from build123d import *

# Parameters (mm, degrees)
SKETCH_1_W      = 38.4
SKETCH_1_H      = 54.1
EXTRUDE_1_DEPTH = 0.8
SKETCH_2_W      = 10
SKETCH_2_H      = 10
EXTRUDE_2_DEPTH = 3


with BuildPart() as part:
    # Эскиз1 → Бобышка-Вытянуть1 (new, symmetric)
    with BuildSketch(Plane(origin=(0, 0, 0), x_dir=(1, 0, 0), z_dir=(0, 1, 0))):
        Rectangle(SKETCH_1_W, SKETCH_1_H)
    extrude(amount=EXTRUDE_1_DEPTH, both=True)

    # Эскиз2 → Бобышка-Вытянуть2 (add)
    with BuildSketch(Plane(origin=(0, 0.8, 0), x_dir=(1, 0, 0), z_dir=(0, 1, 0))):
        with Locations((-14.2, 19.164621175)):
            Rectangle(SKETCH_2_W, SKETCH_2_H)
        with Locations((-14.2, 6.274815906)):
            Rectangle(SKETCH_2_W, SKETCH_2_H)
        with Locations((-14.2, -7.606512846)):
            Rectangle(SKETCH_2_W, SKETCH_2_H)
        with Locations((-14.2, -20.685179731)):
            Rectangle(SKETCH_2_W, SKETCH_2_H)
        with Locations((14.2, 18.692467136)):
            Rectangle(SKETCH_2_W, SKETCH_2_H)
        with Locations((14.2, 5.897092674)):
            Rectangle(SKETCH_2_W, SKETCH_2_H)
        with Locations((14.2, -6.756635575)):
            Rectangle(SKETCH_2_W, SKETCH_2_H)
        with Locations((14.2, -21.110118366)):
            Rectangle(SKETCH_2_W, SKETCH_2_H)
    extrude(amount=EXTRUDE_2_DEPTH)


solid = part.part
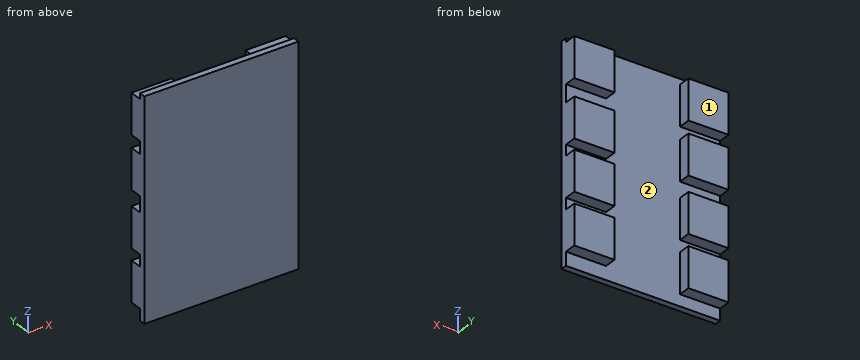
Build history of the part. All positions in model axes, mm. Face numbers are marked on the shaded views. Round coordinates to 2 decimals unless told otherwise and drop trailing zeros. Loops run counter-clockwise (first coordinate to the right, second up) from the corner with the lowest first, then second, coordinate; pieces in that order, holes last. Notation, with made-up numbers: (-24, -18.75) -> (13, -18.75) arc R25 cw to (13, 5.25) -> close; hole circle Ø9 at (37.25, -6). An arc over 180 degrees is marked (long way). One line per item, written item: value. Start each with the question number.
Q1. Drop flat-ended pins along their axis: pin 1 Ø0.9 at (x, y) = (-15.5, 2.5) entering from +Z; pin 2 Ø0.9 at (x, y) = (12, 2) entering from -Z; pin 3 Ø2 at (x, y) = (-10.5, 2.5) entering from -Z. Give the stop position or say it passes through.
Q2. Probe line 1 along Z through (x, y) = (-11.5, 3.2); line 2 along Z through (x, y) = (13.5, 2.9); line 3 along X through (y, z) = (1.9, 24.5). List the from-to ranges inside material, lowest first.
Q3. Cut at B-B on x = 10. List the corners of the cut face in (y, z).
Q4. Cut at A-A on y = 2.9. Count the separate pieces of the cut face and the enclosed holes in it, plus the area to 3 significant figures.
Q5. Two-plate mould, pull along Z, no slides. Class the marked faces 1 and 2: released by +Z, released by -Z, zero draft, split by the parting line, or undercut.
Q6. Cut at C-C on z = 17. List the corners of the cut face in (x, y).
Computed:
1. pin 1: z = 25.69
1. pin 2: z = -23.69
1. pin 3: z = -24.16
2. line 1: -24.16 to -14.16, -11.27 to -1.27, 2.61 to 12.61, 15.69 to 25.69
2. line 2: -23.69 to -13.69, -10.9 to -0.9, 1.76 to 11.76, 16.11 to 26.11
2. line 3: -19.2 to -9.2, 9.2 to 19.2
3. outline: (-0.8, -27.05) -> (0.8, -27.05) -> (0.8, -23.69) -> (3.8, -23.69) -> (3.8, -13.69) -> (0.8, -13.69) -> (0.8, -10.9) -> (3.8, -10.9) -> (3.8, -0.9) -> (0.8, -0.9) -> (0.8, 1.76) -> (3.8, 1.76) -> (3.8, 11.76) -> (0.8, 11.76) -> (0.8, 16.11) -> (3.8, 16.11) -> (3.8, 26.11) -> (0.8, 26.11) -> (0.8, 27.05) -> (-0.8, 27.05) -> close
4. separate pieces: 8
4. enclosed holes: 0
4. area: 800 mm²
5. face 1: zero draft
5. face 2: undercut
6. outline: (-19.2, -0.8) -> (19.2, -0.8) -> (19.2, 3.8) -> (9.2, 3.8) -> (9.2, 0.8) -> (-9.2, 0.8) -> (-9.2, 3.8) -> (-19.2, 3.8) -> close
